```python
from build123d import *

# Parameters (mm, degrees)
SKETCH1_R                = 37.5
BOSS_EXTRUDE1_DEPTH      = 10.16
SKETCH2_R                = 32.081215916
CUT_EXTRUDE1_DEPTH       = 10.16
SKETCH4_R                = 32.081215916
BOSS_EXTRUDE3_DEPTH      = 2.54
BOSS_EXTRUDE3_DEPTH_BACK = 2.54
CUT_EXTRUDE2_DEPTH       = 15.24
SKETCH6_R                = 3.281091855
CUT_EXTRUDE3_DEPTH       = 15.24


with BuildPart() as part:
    # Sketch1 → Boss-Extrude1 (new body)
    with BuildSketch(Plane.XY):
        Circle(SKETCH1_R)
    extrude(amount=BOSS_EXTRUDE1_DEPTH)

    # Sketch2 → Cut-Extrude1 (cut)
    with BuildSketch(Plane.XY.offset(10.16)):
        Circle(SKETCH2_R)
    extrude(amount=-CUT_EXTRUDE1_DEPTH, mode=Mode.SUBTRACT)

    # Sketch4 → Boss-Extrude3 (add, two sides)
    with BuildSketch(Plane.XY.offset(5.08)) as boss_extrude3_sk:
        Circle(SKETCH4_R)
    extrude(amount=BOSS_EXTRUDE3_DEPTH)
    extrude(boss_extrude3_sk.sketch, amount=-BOSS_EXTRUDE3_DEPTH_BACK)

    # Sketch5 → Cut-Extrude2 (cut)
    with BuildSketch(Plane.XY.offset(7.62)):
        with BuildLine():
            Line((-3.738926609, 10.791901804), (-3.738926609, 26.50033006))
            ThreePointArc((-3.738926609, 26.50033006), (-18.924152101, 18.924152101), (-26.50033006, 3.738926609))
            Line((-26.50033006, 3.738926609), (-10.791901804, 3.738926609))
            ThreePointArc((-10.791901804, 3.738926609), (-8.076036055, 8.076036055), (-3.738926609, 10.791901804))
        make_face()
        with BuildLine():
            Line((3.738926609, 10.791901804), (3.738926609, 26.50033006))
            ThreePointArc((3.738926609, 26.50033006), (18.924152101, 18.924152101), (26.50033006, 3.738926609))
            Line((26.50033006, 3.738926609), (10.791901804, 3.738926609))
            ThreePointArc((10.791901804, 3.738926609), (8.076036055, 8.076036055), (3.738926609, 10.791901804))
        make_face()
        with BuildLine():
            Line((10.791901804, -3.738926609), (26.50033006, -3.738926609))
            ThreePointArc((26.50033006, -3.738926609), (18.924152101, -18.924152101), (3.738926609, -26.50033006))
            Line((3.738926609, -26.50033006), (3.738926609, -10.791901804))
            ThreePointArc((3.738926609, -10.791901804), (8.076036055, -8.076036055), (10.791901804, -3.738926609))
        make_face()
        with BuildLine():
            Line((-3.738926609, -10.791901804), (-3.738926609, -26.50033006))
            ThreePointArc((-3.738926609, -26.50033006), (-18.924152101, -18.924152101), (-26.50033006, -3.738926609))
            Line((-26.50033006, -3.738926609), (-10.791901804, -3.738926609))
            ThreePointArc((-10.791901804, -3.738926609), (-8.076036055, -8.076036055), (-3.738926609, -10.791901804))
        make_face()
    extrude(amount=-CUT_EXTRUDE2_DEPTH, mode=Mode.SUBTRACT)

    # Sketch6 → Cut-Extrude3 (cut)
    with BuildSketch(Plane.XY.offset(7.62)):
        Circle(SKETCH6_R)
    extrude(amount=-CUT_EXTRUDE3_DEPTH, mode=Mode.SUBTRACT)


solid = part.part
```
Build history of the part. All positions in model axes, mm. A direction names the side the tool comes from. Round coordinates to 2 decimals unless told otherwise and drop trailing zeros. Order: outer loops, then holes, each group sorted by start corner. A loop starts at its lowest first (then second) coordinate and runs counter-clockwise, first axis right, second up. Notation, with made-up numbers: (48, 58) -> (83, 58) arc R9 cw to (83, 70) -> close; hole circle Ø8 at (60.5, -22). An arc over 180 degrees is marked (long way). Answer in a Markdown table with one row per item.
1) Wall check: L1, parallel to Y at x = 0, z = 2.05; L2, parallel to X at y = -6, z = 7; L3, parallel to X at y = -11, z = 5. Give the ranges that are in metal, low to high.
Values:
| item | result |
|---|---|
| L1 | -37.5 to -32.08, 32.08 to 37.5 |
| L2 | -37.02 to -26.08, -9.72 to 9.72, 26.08 to 37.02 |
| L3 | -35.85 to -24.4, -3.74 to 3.74, 24.4 to 35.85 |
2) Which spindle directions (+Z, -Z, +X, -X, +Y, -Y) get a long thin tool onto all of the face, cutting with end or side? Do faces 3 (the cylindrical face through (-6.95, -31.32, 8.91)), 4 (the cylindrical face through (-6.95, -31.32, 1.29)), 5 (the flat face through (-19, 3.739, 5)). Say none if no direction does.
Values:
| item | result |
|---|---|
| face 3 | +Z |
| face 4 | -Z |
| face 5 | +Z, -Z |
3) Band-saw the part on D-D on y = 24. Give the cut face in (x, z), and give its area (3 significant figures).
Values:
| item | result |
|---|---|
| outline | (-28.81, 0) -> (-21.29, 0) -> (-21.29, 2.54) -> (-11.84, 2.54) -> (-11.84, 7.62) -> (-21.29, 7.62) -> (-21.29, 10.16) -> (-28.81, 10.16) -> close; (-3.74, 2.54) -> (3.74, 2.54) -> (3.74, 7.62) -> (-3.74, 7.62) -> close; (11.84, 2.54) -> (21.29, 2.54) -> (21.29, 0) -> (28.81, 0) -> (28.81, 10.16) -> (21.29, 10.16) -> (21.29, 7.62) -> (11.84, 7.62) -> close |
| area | 287 mm2 |
4) Band-saw the part on C-C on z = 4. Give the cut face in (x, y), and give its area (3 significant figures).
Values:
| item | result |
|---|---|
| outline | circle Ø75 at (0, 0); hole (-26.5, -3.74) arc R26.76 ccw to (-3.74, -26.5) -> (-3.74, -10.79) arc R11.42 cw to (-10.79, -3.74) -> close; hole (-26.5, 3.74) -> (-10.79, 3.74) arc R11.42 cw to (-3.74, 10.79) -> (-3.74, 26.5) arc R26.76 ccw to start; hole circle Ø6.56 at (0, 0); hole (3.74, -26.5) arc R26.76 ccw to (26.5, -3.74) -> (10.79, -3.74) arc R11.42 cw to (3.74, -10.79) -> close; hole (3.74, 10.79) arc R11.42 cw to (10.79, 3.74) -> (26.5, 3.74) arc R26.76 ccw to (3.74, 26.5) -> close |
| area | 3,010 mm2 |
5) Pin check, flat tips, straight feed: P1, Ø2, axis at x = -30, y = 7, coming from the +Z side; P2, Ø2, axis at y = -22.5, z = 6, coming from the +X side; P3, Ø4, axis at y = -25, z = 6.5, coming from the -X side. Stop position of each tip, or through.
Values:
| item | result |
|---|---|
| P1 | z = 7.62 |
| P2 | x = 30.72 |
| P3 | x = -29.62 |
6) Mould opens along Y. For faces 1 (the cylindrical face through (19.094, -18.752, 5.116)), 2 (the cylindrical face through (-8.13, -8.02, 5.12)) say: released by +Y, released by -Y, zero draft, split by the parting line, or undercut.
Values:
| item | result |
|---|---|
| face 1 | undercut |
| face 2 | undercut |
7) Band-saw the part on A-A on x = 0. Give the cut face in (y, z).
Values:
| item | result |
|---|---|
| outline | (-37.5, 0) -> (-32.08, 0) -> (-32.08, 2.54) -> (-3.28, 2.54) -> (-3.28, 7.62) -> (-32.08, 7.62) -> (-32.08, 10.16) -> (-37.5, 10.16) -> close; (3.28, 2.54) -> (32.08, 2.54) -> (32.08, 0) -> (37.5, 0) -> (37.5, 10.16) -> (32.08, 10.16) -> (32.08, 7.62) -> (3.28, 7.62) -> close |
